Design review of the part built by this model. Coordinates are the model's own, in mm. A direction names the side the tool comes from. Give positions to 0.01 mm unless a question says otherwise; leave off trailing zeros. Order: outer loops, then holes, each group sorted by start corner. A loop starts at its lowest first (then second) coordinate and runs counter-clockwise, first axis right, second up.
```python
from build123d import *

# Parameters (mm, degrees)
SKETCH1_W           = 55
SKETCH1_H           = 35
BOSS_EXTRUDE1_DEPTH = 6.35
SKETCH2_R           = 0.79375
BOSS_EXTRUDE2_DEPTH = 6.35
SKETCH4_R           = 1.587499993
CUT_EXTRUDE2_DEPTH  = 0.254
SKETCH5_W           = 52.968
SKETCH5_H           = 32.968
CUT_EXTRUDE3_DEPTH  = 2.54
SKETCH6_W           = 42.808
SKETCH6_H           = 22.808
BOSS_EXTRUDE3_DEPTH = 1.27


with BuildPart() as part:
    # Sketch1 → Boss-Extrude1 (new body)
    with BuildSketch(Plane.XY):
        with Locations((-56.246376812, 16.09057971)):
            Rectangle(SKETCH1_W, SKETCH1_H)
    extrude(amount=BOSS_EXTRUDE1_DEPTH)

    # Sketch2 → Boss-Extrude2 (add)
    with BuildSketch(Plane(origin=(-28.746376812, 0, 0), x_dir=(0, 0, -1), z_dir=(1, 0, 0))):
        with Locations(Location((-3.175, 17.67807971, 0), (0, 0, 270))):
            Circle(SKETCH2_R)
        with Locations(Location((-3.175, 14.50307971, 0), (0, 0, 270))):
            Circle(SKETCH2_R)
    extrude(amount=BOSS_EXTRUDE2_DEPTH)

    # Sketch4 → Cut-Extrude2 (cut)
    with BuildSketch(Plane(origin=(0, 0, 0), x_dir=(-1, 0, 0), z_dir=(0, 0, -1))):
        with Locations((56.246376812, 16.09057971)):
            Circle(SKETCH4_R)
    extrude(amount=-CUT_EXTRUDE2_DEPTH, mode=Mode.SUBTRACT)

    # Sketch5 → Cut-Extrude3 (cut)
    with BuildSketch(Plane.XY.offset(6.35)):
        with Locations((-56.246376812, 16.09057971)):
            Rectangle(SKETCH5_W, SKETCH5_H)
    extrude(amount=-CUT_EXTRUDE3_DEPTH, mode=Mode.SUBTRACT)

    # Sketch6 → Boss-Extrude3 (add)
    with BuildSketch(Plane.XY.offset(3.81)):
        with Locations((-56.246376812, 16.09057971)):
            Rectangle(SKETCH6_W, SKETCH6_H)
    extrude(amount=BOSS_EXTRUDE3_DEPTH)


solid = part.part
```
1. Take a section at A-A (y = 13). State the section outline as (x, z) points, then the cut area to 3 significant figures.
Recorded:
outline: (-83.75, 0) - (-28.75, 0) - (-28.75, 6.35) - (-29.76, 6.35) - (-29.76, 3.81) - (-34.84, 3.81) - (-34.84, 5.08) - (-77.65, 5.08) - (-77.65, 3.81) - (-82.73, 3.81) - (-82.73, 6.35) - (-83.75, 6.35) - close
area: 269 mm2
2. Machinability: for faces 4 (the face through (-57, -1.409, 3)), 5 (the face through (-25.616, 18.308, 3.658)), 6 (the face through (-29.762, 16, 5)), 7 (the face through (-56, 16, 0.254)), 8 (the face through (-22.396, 18, 3)), which of the approach directions +Z, -Z, +X, -X, +Y, -Y give a long, thin tool a straight path to every point of the face, cutting with its end or side? Answer none if there is none.
Recorded:
face 4: +Z, -Z, +X, -X, -Y
face 5: +X
face 6: +Z
face 7: -Z
face 8: +Z, -Z, +X, +Y, -Y
3. Draft analysis for pull direction Y (two halves, no side actions). For faces 1 (the face through (-65, 33, 6.35)), 2 (the face through (-57, 33.591, 3)), 3 (the face through (-34.842, 16, 4)), state which applies: pulls with the +Y half, pulls with the -Y half, needs draft (parallel to the pull), parting line crosses it, or undercut.
Recorded:
face 1: needs draft
face 2: pulls with the +Y half
face 3: undercut
4. For pin 1 (5 mm diameter, centred on x = -56.25, y = 16.09, fed in from +Z); pin 2 (0.8 mm diameter, centred on y = 17, z = 5.5, fed in from +X), all flat-tipped, find the tip position at first contact; note any pin that passes through.
Recorded:
pin 1: stops at z = 5.08
pin 2: stops at x = -28.75
5. Take a section at D-D (x = -50). State the section outline as (y, z) points, then the cut area to 3 significant figures.
Recorded:
outline: (-1.41, 0) - (33.59, 0) - (33.59, 6.35) - (32.57, 6.35) - (32.57, 3.81) - (27.49, 3.81) - (27.49, 5.08) - (4.69, 5.08) - (4.69, 3.81) - (-0.39, 3.81) - (-0.39, 6.35) - (-1.41, 6.35) - close
area: 167 mm2
6. Take a section at C-C (z = 1.25). State the section outline as (x, y) points.
Recorded:
outline: (-83.75, -1.41) - (-28.75, -1.41) - (-28.75, 33.59) - (-83.75, 33.59) - close
7. For line 1 along X through (y, z) = (19.5, 4.5); line 2 along Y through (x, z) = (-36.5, 5); line 3 along Y through (x, z) = (-48.5, 5.25), list the stretches that pass through material, from the lowest coordinate up.
Recorded:
line 1: x = -83.75 to -82.73, -77.65 to -34.84, -29.76 to -28.75
line 2: y = -1.41 to -0.39, 4.69 to 27.49, 32.57 to 33.59
line 3: y = -1.41 to -0.39, 32.57 to 33.59
8. Take a section at B-B (x = -31). State the section outline as (y, z) points, then the cut area to 3 significant figures.
Recorded:
outline: (-1.41, 0) - (33.59, 0) - (33.59, 6.35) - (32.57, 6.35) - (32.57, 3.81) - (-0.39, 3.81) - (-0.39, 6.35) - (-1.41, 6.35) - close
area: 139 mm2
